Check sheet for the modelled part. Datum: model origin and axes. Units: mm. A direction names the side the tool comes from. Coordinates: 2 decimals unless noted, no trailing zeros. Loops run counter-clockwise (first coordinate to the right, second up) from the corner with the lowest first, then second, coordinate; pieces in that order, holes last. Notation, with made-up numbers: (-4.75, -11) -> (30.25, -11) arc R22 ccw to (30.25, 26) -> close; hole circle Ø1 at (-17.75, -5.75). An arc over 180 degrees is marked (long way). Use CSV: the item, a comma, the result in double quotes. Start each with the question number.
1. Sectioned sample at A-A, the plane x = 15. Record the cut outline in (y, z) (3 decimals), and give its area (3 significant figures).
2. Gauge pin test, flat ends, axial feed: pin 1 (6 mm diameter, centred on x = 51.5, y = -1, fed in from +Z); pin 2 (2 mm diameter, centred on x = 30, y = -1, fed in from +Z); pin 3 (2.5 mm diameter, centred on y = 6, z = 2, fed in from -X). Record the tip position at first contact, or that the pin passes through.
3. Sectioned sample at D-D, the plane x = 36.5. Record the cut outline in (y, z).
4. Sectioned sample at B-B, the plane y = 5. Record the cut outline in (x, z) (3 decimals), and give its area (3 significant figures).
5. Set-up check for faces 5 (the face through (58, -1, 8)), 6 (the face through (34, 5, 3)), 7 (the face through (10.25, 5, 2)): record each of +Z, -Z, +X, -X, +Y, -Y from which the full face is reachable in a straight line by a thin tool's end or side.
6. Release check for a two-part mould opening along Y. For faces 1 (the face through (29, -5, 10)), 2 (the face through (34, 10, 1)), 3 (the face through (0, -3, 10)), 4 (the face through (41.377, 5.071, 1.521)) record: pulls with the +Y half, pulls with the -Y half, needs draft (parallel to the pull), parting line crosses it, or undercut.
7. Sectioned sample at C-C, the plane z = 2. Record the cut outline in (x, y) (3 decimals), and give its area (3 significant figures).
8. Thickness scan on L1, parallel to Y at x = 15, z = 1.2 (3 decimals); L2, parallel to Y at x = 36, z = 13.25; L3, parallel to Z at x = 48.5, y = 2.25. Record the ranges inside material, lowest first.
```python
from build123d import *

# Parameters (mm, degrees)
ESQUISSE1_W             = 58
ESQUISSE1_H             = 5
BOSS_EXTRU_1_DEPTH      = 20
ESQUISSE3_W             = 47.75
ESQUISSE3_H             = 3
BOSS_EXTRU_2_DEPTH      = 10
ESQUISSE4_R             = 1.625
ENL_V_MAT_EXTRU_1_DEPTH = 10
ENL_V_MAT_EXTRU_2_DEPTH = 59


with BuildPart() as part:
    # Esquisse1 → Boss.-Extru.1 (new body)
    with BuildSketch(Plane.XY):
        with Locations((29, -2.5)):
            Rectangle(ESQUISSE1_W, ESQUISSE1_H)
    extrude(amount=BOSS_EXTRU_1_DEPTH)

    # Esquisse3 → Boss.-Extru.2 (add)
    with BuildSketch(Plane(origin=(0, 0, 0), x_dir=(1, 0, 0), z_dir=(0, 1, 0))):
        with Locations((34.125, -1.5)):
            Rectangle(ESQUISSE3_W, ESQUISSE3_H)
    extrude(amount=BOSS_EXTRU_2_DEPTH)

    # Esquisse4 → Enlèv. mat.-Extru.1 (cut)
    with BuildSketch(Plane.XY.offset(3)):
        with Locations((43, 5)):
            Circle(ESQUISSE4_R)
        with Locations((15, 5)):
            Circle(ESQUISSE4_R)
    extrude(amount=-ENL_V_MAT_EXTRU_1_DEPTH, mode=Mode.SUBTRACT)

    # Esquisse6 → Enlèv. mat.-Extru.2 (cut, through all)
    with BuildSketch(Plane(origin=(58, 0, 0), x_dir=(0, 0, -1), z_dir=(1, 0, 0))):
        Polygon((-20, -5), (-19.75, 0), (-20, 0), align=None)
    extrude(amount=-ENL_V_MAT_EXTRU_2_DEPTH, mode=Mode.SUBTRACT)


solid = part.part
```
Completed:
1,outline,"(-5, 0) -> (3.375, 0) -> (3.375, 3) -> (0, 3) -> (0, 19.75) -> (-5, 20) -> close; (6.625, 0) -> (10, 0) -> (10, 3) -> (6.625, 3) -> close"
1,area,"120 mm²"
2,pin 1,"z = 19.95"
2,pin 2,"z = 19.85"
2,pin 3,"x = 10.25"
3,outline,"(-5, 0) -> (10, 0) -> (10, 3) -> (0, 3) -> (0, 19.75) -> (-5, 20) -> close"
4,outline,"(10.25, 0) -> (13.375, 0) -> (13.375, 3) -> (10.25, 3) -> close; (16.625, 0) -> (41.375, 0) -> (41.375, 3) -> (16.625, 3) -> close; (44.625, 0) -> (58, 0) -> (58, 3) -> (44.625, 3) -> close"
4,area,"124 mm²"
5,face 5,"+Z, -Z, +X, +Y, -Y"
5,face 6,"+Z, +X, -X, +Y"
5,face 7,"+Z, -Z, -X, +Y"
6,face 1,"pulls with the -Y half"
6,face 2,"pulls with the +Y half"
6,face 3,"needs draft"
6,face 4,"undercut"
7,outline,"(0, -5) -> (58, -5) -> (58, 10) -> (10.25, 10) -> (10.25, 0) -> (0, 0) -> close; hole circle Ø3.25 at (15, 5); hole circle Ø3.25 at (43, 5)"
7,area,"751 mm²"
8,L1,"-5 to 3.375, 6.625 to 10"
8,L2,"-5 to 0"
8,L3,"0 to 3"
